Check sheet for the modelled part. Datum: model origin and axes. Units: mm. A direction names the side the tool comes from. Coordinates: 2 decimals unless noted, no trailing zeros. Loops run counter-clockwise (first coordinate to the right, second up) from the corner with the lowest first, then second, coordinate; pieces in that order, holes last. Notation, with made-up numbers: (85.25, -35) - (121.25, -35) arc R22 cw to (121.25, -20) - close; hole circle Ø4 at (82.5, -17). An arc over 180 degrees is marked (long way). Write each question's results on one line, items separated by ' | '. Start each with the question number.
1. Cross-section at A-A (z = -2.5). Record the cut outline in (x, y) (3 decimals), and give its area (3 significant figures).
2. Cross-section at D-D (z = -6.5). Record the cut outline in (x, y), and give its area (3 significant figures).
3. Draft check along Y on faces 4 (the face through (8.31, 0.37, -1.52)), 5 (the face through (-5, -16, 6.8)), 6 (the face through (-15.42, -0.68, -1.3)). Enter one of: released by +Y, released by -Y, zero draft, split by the parting line, or undercut.
4. Thickness scan on line 1 (Y direction, x = 0, z = -1.5) (3 decimals); line 2 (Y direction, x = -2, z = -2.5); line 3 (Z direction, x = -0.5, y = 5). Record the ranges inside material, lowest first. Write a range as [from, to].
5. Tool access check on faces 1 (the face through (11, -11, 1)), 2 (the face through (0, 0, 0)), 3 (the face through (4, -4, -3)). Record the directions out of +Z, -Z, +X, -X, +Y, -Y that give a thin tool (end or side, any length) a straight path to the whole face; none if there is none.
6. Cross-section at B-B (x = -9.5). Give the number of separate pieces and of enclosed holes in the cut face, and give its area (3 significant figures).
7. Gauge pin test, flat ends, axial feed: P1, Ø2, axis at x = 11, y = 9.5, coming from the -Z side; P2, Ø3, axis at x = -9.5, y = 0, coming from the -Z side; P3, Ø4, axis at y = -10, z = -4, coming from the +X side; P4, Ø1.5, axis at x = 9.5, y = 0, coming from the +Z side. Record the tip position at first contact, or that the pin passes through.
```python
from build123d import *

# Parameters (mm, degrees)
SKETCH_2_R          = 1.245
SKETCH_2_R_2        = 10.5
CUT_EXTRUDE_1_DEPTH = 4
SKETCH_3_R          = 10.5
CUT_EXTRUDE_2_DEPTH = 2


with BuildPart() as part:
    # Эскиз1 → Повернуть1 (revolve)
    with BuildSketch(Plane(origin=(0, 0, 0), x_dir=(0, 0, -1), z_dir=(1, 0, 0)), mode=Mode.PRIVATE) as revolve_1_sk:
        Polygon((0, 0), (8, 0), (8, 4.75), (3, 4.75), (3, 15), (-6.8, 17.5), (-6.8, 16.5), (0, 14.765306122), align=None)
    revolve(revolve_1_sk.sketch.rotate(Axis((0, 0, 0), (0, 0, -1)), 90), axis=Axis((0, 0, 0), (0, 0, -1)))

    # Эскиз2 → Вырез-Вытянуть1 (cut)
    with BuildSketch(Plane(origin=(0, 0, -3), x_dir=(-1, 0, 0), z_dir=(0, 0, -1))):
        with Locations((0, 8)):
            Circle(SKETCH_2_R)
        with Locations((0, -8)):
            Circle(SKETCH_2_R)
        with Locations((9.5, 0)):
            Circle(SKETCH_2_R)
        with Locations((-9.5, 0)):
            Circle(SKETCH_2_R)
        with Locations((-15.202795796, -15.202795796)):
            Circle(SKETCH_2_R_2)
        with Locations((-15.202795796, 15.202795796)):
            Circle(SKETCH_2_R_2)
        with Locations((15.202795796, -15.202795796)):
            Circle(SKETCH_2_R_2)
    extrude(amount=-CUT_EXTRUDE_1_DEPTH, mode=Mode.SUBTRACT)

    # Эскиз3 → Вырез-Вытянуть2 (cut)
    with BuildSketch(Plane(origin=(0, 0, -3), x_dir=(-1, 0, 0), z_dir=(0, 0, -1))):
        with Locations((15.202795796, 15.202795796)):
            Circle(SKETCH_3_R)
    extrude(amount=-CUT_EXTRUDE_2_DEPTH, mode=Mode.SUBTRACT)


solid = part.part
```
Established:
1) outline: (-14.367, -4.736) arc R10.5 cw to (-4.736, -14.367) arc R15.128 ccw to (4.736, -14.367) arc R10.5 cw to (14.367, -4.736) arc R15.128 ccw to (14.367, 4.736) arc R10.5 cw to (4.736, 14.367) arc R15.128 ccw to (-4.736, 14.367) arc R10.5 cw to (-14.367, 4.736) arc R15.128 ccw to start; hole circle Ø2.49 at (-9.5, 0); hole circle Ø2.49 at (0, -8); hole circle Ø2.49 at (0, 8); hole circle Ø2.49 at (9.5, 0) | area: 546 mm^2
2) outline: circle Ø9.5 at (0, 0) | area: 70.9 mm^2
3) face 4: undercut | face 5: zero draft | face 6: split by the parting line
4) line 1: [-15.383, -9.245], [-6.755, 6.755], [9.245, 15.383] | line 2: [-14.99, 14.99] | line 3: [-3, 0]
5) face 1: -Z, +X, -Y | face 2: +Z | face 3: -Z
6) separate pieces: 3 | enclosed holes: 0 | area: 52.5 mm^2
7) P1: z = 1 | P2: z = -3 | P3: x = 7.32 | P4: through
